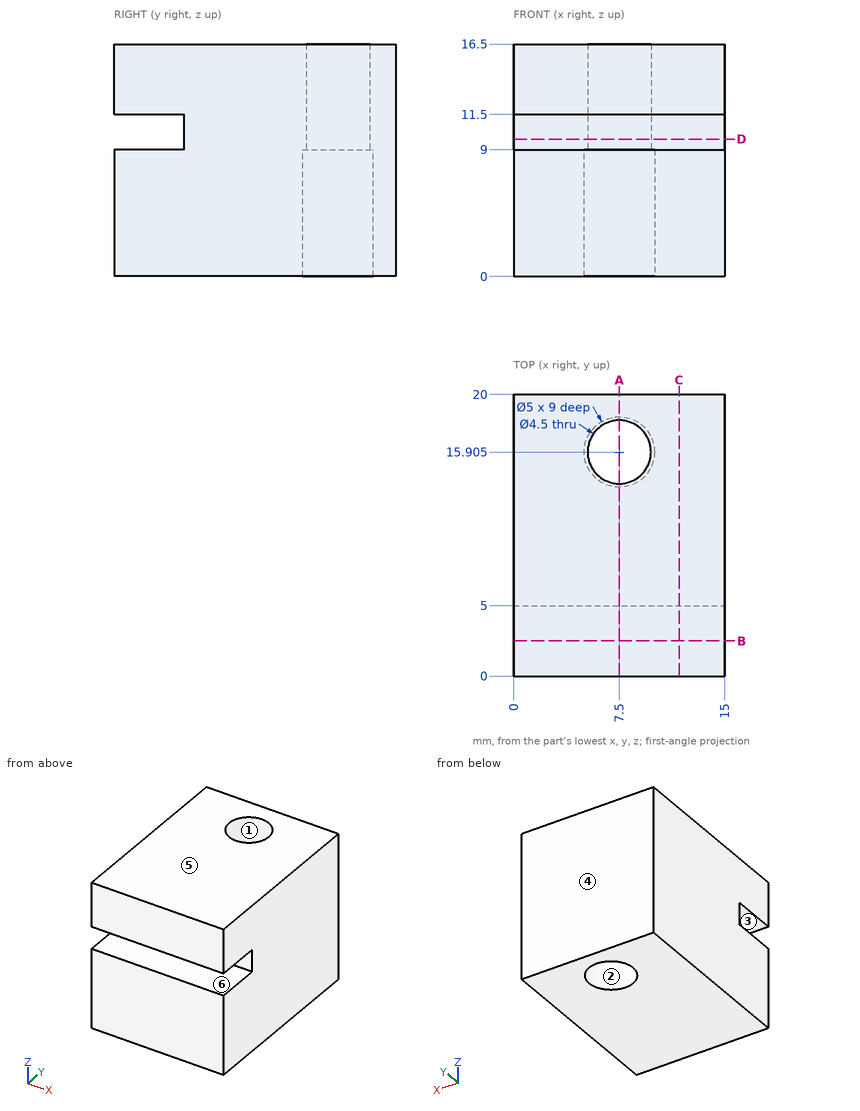
Design review of the part shown in the three views and the two pictorial views. Dimensions are in mm from the part's minimum x, y and z. A direction names the side the tool comes from. Round coordinates to 2 decimals unless told otherwise and drop trailing zeros. Write each loop counter-clockwise with the first axis right and the second up, starting at its lowest first coordinate (ties: lowest second). Pieces come first, ordered by that corner, then holes. Notation, with made-up numbers: (44.5, 75.5) - (55.5, 75.5) arc R23 ccw to (55.5, 108.5) - close; hole circle Ø5 at (11, 56). An arc over 180 degrees is marked (long way). Write item = value, one per line. Start each with the question number.
1. Consider section D-D on z = 9.75. State the section outline as (x, y) points (3 decimals), plus the area to 3 significant figures.
2. For the marked faces 1, 2 and 3, list the 3-axis set-ups (+Z, -Z, +X, -X, +Y, -Y) from which the entire face can be reached by the end or side of a thin tool; tool diameter is ignored.
3. Consider section A-A on x = 7.5. State the section outline as (y, z) points (3 decimals).
4. Consider section B-B on y = 2.5. State the section outline as (x, z) points, plus the area to 3 significant figures.
5. Consider section C-C on x = 11.75. State the section outline as (y, z) points.
6. Wall thickness on L1, parallel to Y at x = 7.5, z = 4.25 (3 decimals); L2, parallel to Y at x = 7.5, z = 15.25 (3 decimals); L3, parallel to Z at x = 11.25, y = 3.25: over which ranges is each line inside the solid? List them lowest first.
7. For pin 1 Ø1.5 at (x, y) = (7.5, 15.5) entering from -Z, flat-tipped, find the tip position at first contact; note if it passes through.
8. Draft analysis for pull direction Z (two halves, no side actions). For the marked faces 4, 5 and 6, state which applies: released by +Z, released by -Z, zero draft, split by the parting line, or undercut.
Evaluation:
q1.outline = (0, 5) - (15, 5) - (15, 20) - (0, 20) - close; hole circle Ø4.5 at (7.5, 15.905)
q1.area = 209 mm2
q2.face_1 = +Z, -Z
q2.face_2 = -Z
q2.face_3 = +X, -X, -Y
q3.outline = (0, 0) - (13.405, 0) - (13.405, 9) - (13.655, 9) - (13.655, 16.5) - (0, 16.5) - (0, 11.5) - (5, 11.5) - (5, 9) - (0, 9) - close; (18.155, 9) - (18.405, 9) - (18.405, 0) - (20, 0) - (20, 16.5) - (18.155, 16.5) - close
q4.outline = (0, 0) - (15, 0) - (15, 9) - (0, 9) - close; (0, 11.5) - (15, 11.5) - (15, 16.5) - (0, 16.5) - close
q4.area = 210 mm2
q5.outline = (0, 0) - (20, 0) - (20, 16.5) - (0, 16.5) - (0, 11.5) - (5, 11.5) - (5, 9) - (0, 9) - close
q6.L1 = 0 to 13.405, 18.405 to 20
q6.L2 = 0 to 13.655, 18.155 to 20
q6.L3 = 0 to 9, 11.5 to 16.5
q7.pin_1 = through
q8.face_4 = zero draft
q8.face_5 = released by +Z
q8.face_6 = undercut
